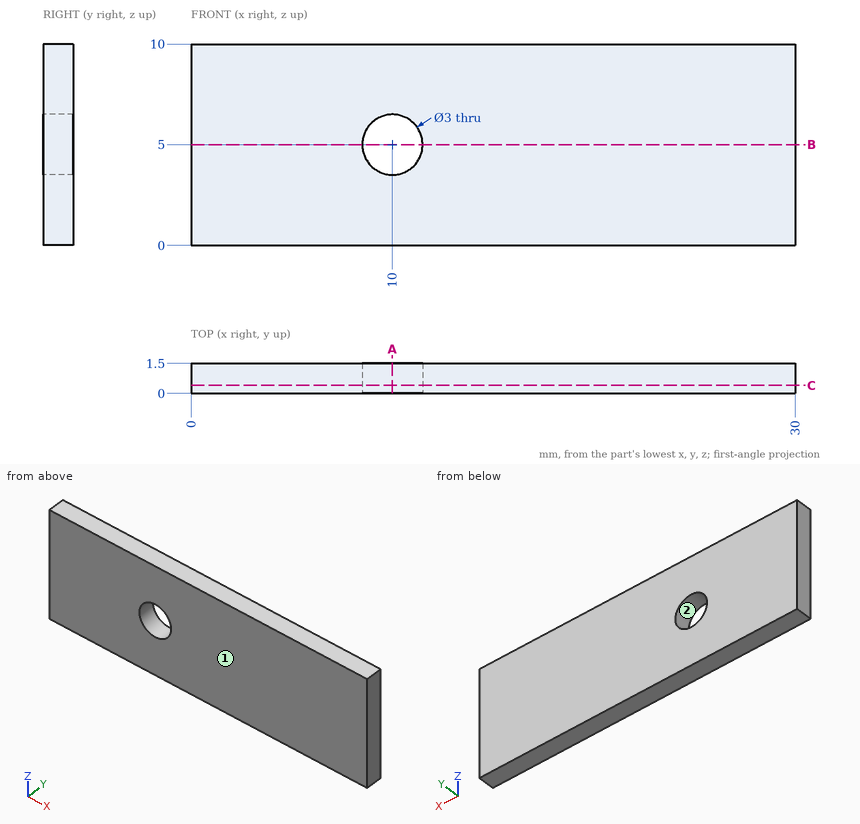
Check sheet for the drawn part. Datum: minimum x, y, z corner. Units: mm. Give positions to 0.01 mm unless a question says otherwise; leave off trailing zeros. Loops run counter-clockwise (first coordinate to the right, second up) from the corner with the lowest first, then second, coordinate; pieces in that order, holes last. Notation, with made-up numbers: (74, 69) - (94, 69) arc R9 cw to (94, 84) - close; hole circle Ø6 at (-37.5, 81). An arc over 180 degrees is marked (long way). Write each question's results on one line, items separated by ' | '.
1) Sectioned sample at B-B on z = 5. Record the boundary of the cut face in (x, y), plus the area to 3 significant figures.
Solution:
outline: (0, 0) - (8.5, 0) - (8.5, 1.5) - (0, 1.5) - close; (11.5, 0) - (30, 0) - (30, 1.5) - (11.5, 1.5) - close | area: 40.5 mm2
2) Sectioned sample at C-C on y = 0.4. Record the boundary of the cut face in (x, z), plus the area to 3 significant figures.
Solution:
outline: (0, 0) - (30, 0) - (30, 10) - (0, 10) - close; hole circle Ø3 at (10, 5) | area: 293 mm2
3) Depth check by flat-ended pin: P1, Ø2.5, axis at x = 10, z = 5, coming from the -Y side. Enter the tip coordinate at first touch or a pass-through.
Solution:
P1: through
4) Material ranges on L1, parallel to Z at x = 10, y = 0.7; L2, parallel to X at y = 0.75, z = 5, recorded low to high. Write a range as from..to.
Solution:
L1: 0..3.5, 6.5..10 | L2: 0..8.5, 11.5..30
5) Sectioned sample at A-A on x = 10. Record the boundary of the cut face in (y, z), plus the area to 3 significant figures.
Solution:
outline: (0, 0) - (1.5, 0) - (1.5, 3.5) - (0, 3.5) - close; (0, 6.5) - (1.5, 6.5) - (1.5, 10) - (0, 10) - close | area: 10.5 mm2
6) Mould release check, pull along Z, two halves, no side actions. Record for the marked faces 1 and 2: pulls with the +Z half, pulls with the -Z half, needs draft (parallel to the pull), parting line crosses it, or undercut.
Solution:
face 1: needs draft | face 2: undercut
